```python
from build123d import *

# Parameters (mm, degrees)
SKETCH1_W           = 48.4
SKETCH1_H           = 38
BOSS_EXTRUDE1_DEPTH = 8
SKETCH2_R           = 3
CUT_EXTRUDE1_DEPTH  = 3
SKETCH3_R           = 1.6
CUT_EXTRUDE2_DEPTH  = 32
CUT_EXTRUDE3_DEPTH  = 3
CUT_EXTRUDE4_DEPTH  = 3
SKETCH6_R           = 1.1
CUT_EXTRUDE5_DEPTH  = 5
CHAMFER1_SIZE       = 0.6
CHAMFER2_SIZE       = 0.5
CHAMFER3_SIZE       = 1.6
SKETCH8_R           = 6
BOSS_EXTRUDE2_DEPTH = 8
CHAMFER4_SIZE       = 2
CHAMFER5_SIZE       = 0.6


with BuildPart() as part:
    # Sketch1 → Boss-Extrude1 (new body)
    with BuildSketch(Plane.XY):
        with Locations((-5.2, 0)):
            Rectangle(SKETCH1_W, SKETCH1_H)
        with BuildLine():
            Line((-7, 12.124355653), (0, 16.165807537))
            Line((0, 16.165807537), (7, 12.124355653))
            ThreePointArc((7, 12.124355653), (14, 0), (7, -12.124355653))
            Line((7, -12.124355653), (0, -16.165807537))
            Line((0, -16.165807537), (-7, -12.124355653))
            ThreePointArc((-7, -12.124355653), (-14, 0), (-7, 12.124355653))
        make_face(mode=Mode.SUBTRACT)
        with BuildLine():
            Line((-15.8, -12.614359354), (-15, -12.152479139))
            Line((-15, -12.152479139), (-14.2, -12.614359354))
            ThreePointArc((-14.2, -12.614359354), (-13.4, -14), (-14.2, -15.385640646))
            Line((-14.2, -15.385640646), (-15, -15.847520861))
            Line((-15, -15.847520861), (-15.8, -15.385640646))
            ThreePointArc((-15.8, -15.385640646), (-16.6, -14), (-15.8, -12.614359354))
        make_face(mode=Mode.SUBTRACT)
    extrude(amount=BOSS_EXTRUDE1_DEPTH)

    # Sketch2 → Cut-Extrude1 (cut)
    with BuildSketch(Plane(origin=(0, 19, 0), x_dir=(1, 0, 0), z_dir=(0, 1, 0))):
        with Locations(Location((-23.2, -4, 0), (0, 0, 270))):
            Circle(SKETCH2_R)
    extrude(amount=-CUT_EXTRUDE1_DEPTH, mode=Mode.SUBTRACT)

    # Sketch3 → Cut-Extrude2 (cut)
    with BuildSketch(Plane(origin=(0, 16, 0), x_dir=(1, 0, 0), z_dir=(0, 1, 0))):
        with Locations(Location((-23.2, -4, 0), (0, 0, 270))):
            Circle(SKETCH3_R)
    extrude(amount=-CUT_EXTRUDE2_DEPTH, mode=Mode.SUBTRACT)

    # Sketch4 → Cut-Extrude3 (cut)
    with BuildSketch(Plane.XZ.offset(19)):
        Polygon((-25.95, 5.58771324), (-25.95, 2.41228676), (-23.2, 0.824573519), (-20.45, 2.41228676), (-20.45, 5.58771324), (-23.2, 7.175426481), align=None)
    extrude(amount=-CUT_EXTRUDE3_DEPTH, mode=Mode.SUBTRACT)

    # Sketch5 → Cut-Extrude4 (cut)
    with BuildSketch(Plane(origin=(0, 0, 0), x_dir=(-1, 0, 0), z_dir=(0, 0, -1))):
        Polygon((12.25, -15.58771324), (12.25, -12.41228676), (15, -10.824573519), (17.75, -12.41228676), (17.75, -15.58771324), (15, -17.175426481), align=None)
    extrude(amount=-CUT_EXTRUDE4_DEPTH, mode=Mode.SUBTRACT)

    # Sketch6 → Cut-Extrude5 (cut)
    with BuildSketch(Plane(origin=(0, 19, 0), x_dir=(1, 0, 0), z_dir=(0, 1, 0))):
        with Locations(Location((-15.1, -4, 0), (0, 0, 270))):
            Circle(SKETCH6_R)
    extrude(amount=-CUT_EXTRUDE5_DEPTH, mode=Mode.SUBTRACT)

    # Chamfer1
    chamfer1_edges = [part.edges().sort_by_distance(p)[0] for p in [
        (-15.1, 19, 2.9),
        (-24.575, -19, 6.38156986),
        (-25.95, -19, 4),
        (-24.575, -19, 1.61843014),
        (-21.825, -19, 1.61843014),
        (-20.45, -19, 4),
        (-21.825, -19, 6.38156986),
    ]]
    chamfer(chamfer1_edges, length=CHAMFER1_SIZE)

    # Chamfer2
    chamfer2_edges = [part.edges().sort_by_distance(p)[0] for p in [
        (-14, 0, 8),
        (-3.5, -14.145081595, 8),
        (3.5, -14.145081595, 8),
        (14, 0, 8),
        (3.5, 14.145081595, 8),
        (-3.5, 14.145081595, 8),
    ]]
    chamfer(chamfer2_edges, length=CHAMFER2_SIZE)

    # Chamfer3
    # the kernel refuses this chamfer: 1.6 mm, written as the material it takes off along each edge
    with BuildSketch(Plane(origin=(-23.2, -16, 4), x_dir=(0, 0, 1), z_dir=(-1, 0, 0))) as chamfer3_piece_1_section:
        Polygon((1.6, CHAMFER3_SIZE), (1.6 + CHAMFER3_SIZE, 0), (1.6, 0), align=None)
    chamfer3_piece_1 = revolve(axis=Axis((-23.2, -16, 4), (0, 1, 0)), mode=Mode.PRIVATE)
    chamfer3_piece_1 = split(chamfer3_piece_1, bisect_by=Plane(origin=(-25.591184435, -15.183394219, 5.794875504), z_dir=(0.5000000000000009, 0, -0.8660254037844382)), keep=Keep.TOP, mode=Mode.PRIVATE)
    chamfer3_piece_1 = split(chamfer3_piece_1, bisect_by=Plane(origin=(-20.808815565, -15.183394219, 5.794875504), z_dir=(-0.4999999999999998, 0, -0.8660254037844388)), keep=Keep.TOP, mode=Mode.PRIVATE)
    chamfer3_piece_1 = split(chamfer3_piece_1, bisect_by=Plane(origin=(-25.95, -15.183394219, 1.653222572), z_dir=(1, 0, 0)), keep=Keep.TOP, mode=Mode.PRIVATE)
    chamfer3_piece_1 = split(chamfer3_piece_1, bisect_by=Plane(origin=(-20.45, -15.183394219, 1.653222572), z_dir=(-1, 0, 0)), keep=Keep.TOP, mode=Mode.PRIVATE)
    chamfer3_piece_1 = split(chamfer3_piece_1, bisect_by=Plane(origin=(-23.558815565, -15.183394219, 1.031735783), z_dir=(0.5000000000000006, 0, 0.8660254037844384)), keep=Keep.TOP, mode=Mode.PRIVATE)
    chamfer3_piece_1 = split(chamfer3_piece_1, bisect_by=Plane(origin=(-22.841184435, -15.183394219, 1.031735783), z_dir=(-0.4999999999999998, 0, 0.8660254037844388)), keep=Keep.TOP, mode=Mode.PRIVATE)
    add(chamfer3_piece_1, mode=Mode.SUBTRACT)

    # Sketch8 → Boss-Extrude2 (add)
    with BuildSketch(Plane(origin=(0, 19, 0), x_dir=(1, 0, 0), z_dir=(0, 1, 0))):
        with Locations(Location((13, -4, 0), (0, 0, 138.189685104))):
            Circle(SKETCH8_R)
    extrude(amount=BOSS_EXTRUDE2_DEPTH)

    # Chamfer4
    # the kernel refuses this chamfer: 2 mm, written as the material it adds along each edge
    with BuildSketch(Plane(origin=(22.615501931, 19, 0), x_dir=(0, -0.9996219169112968, 0.02749587661058639), z_dir=(-1, 0, 0))) as chamfer4_piece_1_section:
        Polygon((CHAMFER4_SIZE * 0.999621916911, -CHAMFER4_SIZE * 0.0274958766106), (-CHAMFER4_SIZE * 0.0274958766106, -CHAMFER4_SIZE * 0.999621916911), (0, 0), align=None)
    chamfer4_piece_1 = extrude(amount=19.231003862, mode=Mode.PRIVATE)
    chamfer4_piece_1 = chamfer4_piece_1 & Plane(origin=(13, 18.289975825, 4), x_dir=(-0.7453559924973536, 0, -0.666666666669547), z_dir=(0, -1, 0)) * Cylinder(6, 47, mode=Mode.PRIVATE)
    add(chamfer4_piece_1)
    with BuildSketch(Plane(origin=(22.615501931, 19, 8), x_dir=(0, -0.9996219169112968, -0.02749587661058651), z_dir=(-1, 0, 0))) as chamfer4_piece_2_section:
        Polygon((CHAMFER4_SIZE * 0.999621916911, CHAMFER4_SIZE * 0.0274958766106), (-CHAMFER4_SIZE * 0.0274958766106, CHAMFER4_SIZE * 0.999621916911), (0, 0), align=None)
    chamfer4_piece_2 = extrude(amount=19.231003862, mode=Mode.PRIVATE)
    chamfer4_piece_2 = chamfer4_piece_2 & Plane(origin=(13, 18.289975825, 4), x_dir=(-0.7453559924973536, 0, -0.666666666669547), z_dir=(0, -1, 0)) * Cylinder(6, 47, mode=Mode.PRIVATE)
    add(chamfer4_piece_2)

    # Chamfer5
    chamfer5_edges = [part.edges().sort_by_distance(p)[0] for p in [
        (17.472135955, 27, 8),
    ]]
    chamfer(chamfer5_edges, length=CHAMFER5_SIZE)


solid = part.part
```
Build history of the part. All positions in model axes, mm. A direction names the side the tool comes from. Give positions to 0.01 mm unless a question says otherwise; leave off trailing zeros. Loops run counter-clockwise (first coordinate to the right, second up) from the corner with the lowest first, then second, coordinate; pieces in that order, holes last.
1) Probe line 1 along X through (y, z) = (18.35, 4); line 2 along X through (y, z) = (15.3, 4); line 3 along X through (y, z) = (12, 2.75). List the from-to ranges inside material, lowest first.
Values follow:
line 1: x = -29.4 to -26.2, -20.2 to -16.2, -14 to 19
line 2: x = -29.4 to -24.8, -21.6 to -16.2, -14 to -1.5, 1.5 to 19
line 3: x = -29.4 to -24.2, -22.2 to -7.21, 7.21 to 19
2) Band-saw the part on B-B on y = 22. List the corners of the cut face in (x, z), then the cut area to 3 significant figures.
Values follow:
outline: circle Ø12 at (13, 4)
area: 113 mm2
3) 3-axis set-ups, long thin cutter, end or side, ignore diameter. For faces 4 (the face through (-25.95, -17, 4)), 5 (the face through (-14, 0, 4)), 6 (the face through (-3.549, 14.401, 7.746)), 7 (the face through (-16.076, 16.231, 4.508)): which of +Z, -Z, +X, -X, +Y, -Y reach the whole face in a straight line?
Values follow:
face 4: -Y
face 5: +Z, -Z
face 6: +Z
face 7: +Y
4) Drop flat-ended pins along their axis: P1, Ø3, axis at x = -15.5, y = -15, coming from the -Z side; P2, Ø1.8, axis at x = -15.5, z = 4, coming from the +Y side; P3, Ø4, axis at x = -18.5, z = 0.5, coming from the +Y side. Give the stop position or say it passes through.
Values follow:
P1: stops at z = 3
P2: stops at y = 18.6
P3: stops at y = 19
5) Band-saw the part on A-A on x = -3. List the corners of the cut face in (y, z).
Values follow:
outline: (-19, 0) - (-14.43, 0) - (-14.43, 7.5) - (-15.01, 8) - (-19, 8) - close; (14.43, 0) - (19, 0) - (19, 8) - (15.01, 8) - (14.43, 7.5) - close
6) Band-saw the part on C-C on y = 10.5. State how many separate pieces and enclosed holes the cut face has, then the cut area to 3 significant figures.
Values follow:
separate pieces: 2
enclosed holes: 1
area: 231 mm2
7) Two-plate mould, pull along Y, no slides. Class faces 1 (the face through (-17.75, -14, 1)), 2 (the face through (18.5, 19, 7)), 3 (the face through (13, 18, -1)): released by +Y, released by -Y, zero draft, split by the parting line, or undercut.
Values follow:
face 1: undercut
face 2: released by +Y
face 3: released by -Y
